Geometry: see drawing. Coordinates: mm, zero at the bounding-box minimum. Give positions to 0.01 mm unless a question says otherwise; leave off trailing zeros. Loops run counter-clockwise (first coordinate to the right, second up) from the corner with the lowest first, then second, coordinate; pieces in that order, holes last. Notation, with made-up numbers: M 15.5,60 L 50.5,60 A33 cw 50.5,95 Z; hole C 82,57 d1. An arc over 180 degrees is marked long. Return JSON: item names as keys, results as strings. Group by question number.
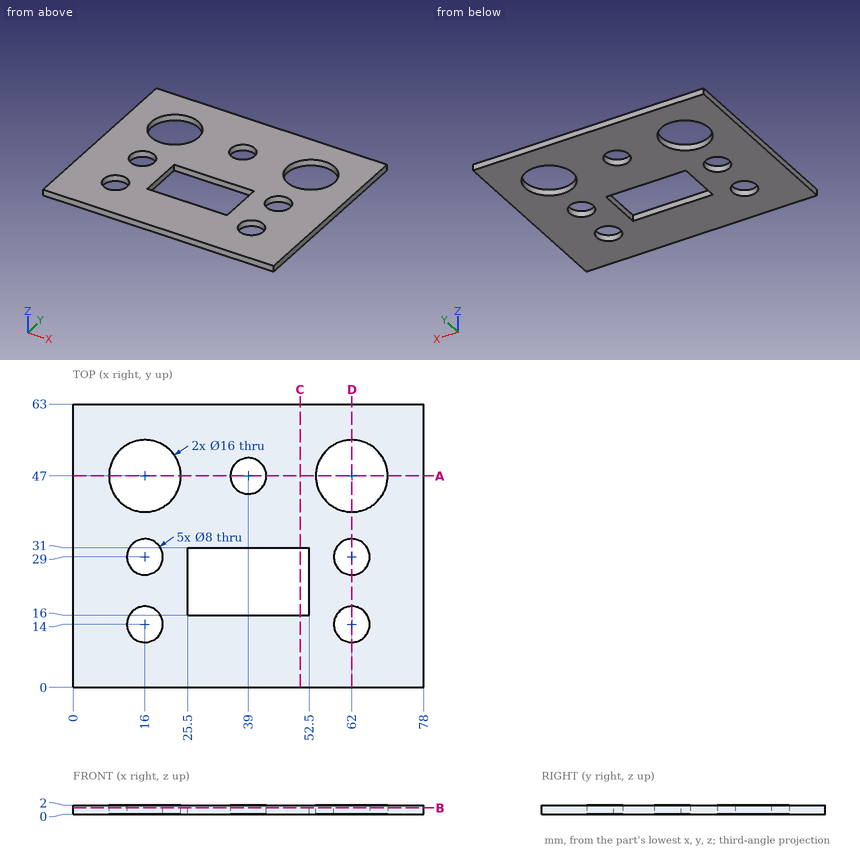
Item 1: Section A-A, the plane y = 47. Return loops of the section in (x, z).
Item 2: Section C-C, the plane x = 50.5. Return loops of the section in (y, z).
Item 3: First-contact query: pin 1 Ø8 at (x, y) = (23, 6.5) entering from -Z. Flat tip, straight axial feed; report the tip coordinate or a pass-through.
Item 4: Section D-D, the plane x = 62. Return loops of the section in (y, z), then the cut area to 3 significant figures.
Item 5: Material intervals for line 1 (Y direction, x = 16, z = 0.6); line 2 (Y direction, x = 15, z = 0.45); line 3 (X direction, y = 26.5, z = 1.4), sorted ascending. Write a range as from..to.
Item 6: Section B-B, the plane z = 1.4. Give the number of separate pieces and of enclosed holes in the cut face, then the cut area to 3 significant figures.
Answer below:
{
 "1": {"outline": "M 0,0 L 8,0 L 8,2 L 0,2 Z; M 24,0 L 35,0 L 35,2 L 24,2 Z; M 43,0 L 54,0 L 54,2 L 43,2 Z; M 70,0 L 78,0 L 78,2 L 70,2 Z"},
 "2": {"outline": "M 0,0 L 16,0 L 16,2 L 0,2 Z; M 31,0 L 63,0 L 63,2 L 31,2 Z"},
 "3": {"pin 1": "z = 0"},
 "4": {"outline": "M 0,0 L 10,0 L 10,2 L 0,2 Z; M 18,0 L 25,0 L 25,2 L 18,2 Z; M 33,0 L 39,0 L 39,2 L 33,2 Z; M 55,0 L 63,0 L 63,2 L 55,2 Z", "area": "62.0 mm^2"},
 "5": {"line 1": "0..10, 18..25, 33..39, 55..63", "line 2": "0..10.13, 17.87..25.13, 32.87..39.06, 54.94..63", "line 3": "0..12.88, 19.12..25.5, 52.5..58.88, 65.12..78"},
 "6": {"separate pieces": "1", "enclosed holes": "8", "area": "3,860 mm^2"}
}
